```python
from build123d import *

# Parameters (mm, degrees)
SKETCH001_R   = 2.5
SKETCH001_R_2 = 8
PAD_DEPTH     = 1
SKETCH003_R   = 4
PAD001_DEPTH  = 9
SKETCH004_R   = 1.3
POCKET_DEPTH  = 9
FILLET_R      = 10
FILLET001_R   = 15
FILLET002_R   = 30
FILLET003_R   = 10
FILLET004_R   = 10
FILLET005_R   = 5


with BuildPart() as part:
    # Sketch001 → Pad (new body)
    with BuildSketch(Plane.XY):
        Polygon((43.04995, 229.318703), (43.04995, 179.449575), (-116.95005, 179.449575), (-116.95005, 239.449575), (-101.796377, 239.449575), (-91.665504, 229.318703), align=None)
        with Locations((5.54995, 200.560838)):
            Circle(SKETCH001_R, mode=Mode.SUBTRACT)
        with Locations((-99.039165, 191.452072)):
            Circle(SKETCH001_R_2, mode=Mode.SUBTRACT)
        with Locations((30.960835, 191.452072)):
            Circle(SKETCH001_R_2, mode=Mode.SUBTRACT)
        with BuildLine():
            ThreePointArc((25.54995, 206.028969), (20.061493, 220.835101), (5.54995, 227.060838))
            Line((-1.19441, 227.060838), (5.54995, 227.060838))
            Line((-9.694456, 218.560838), (-1.19441, 227.060838))
            Line((-113.95005, 218.561117), (-9.694456, 218.560838))
            Line((-113.95005, 218.561117), (-113.95005, 209.560838))
            Line((-113.95005, 209.560838), (-9.618024, 209.560838))
            Line((-9.618024, 209.560838), (5.54995, 209.560838))
            Line((5.54995, 209.560838), (10.697892, 204.412896))
            Line((10.697892, 189.560838), (10.697892, 204.412896))
            ThreePointArc((10.697892, 189.560838), (21.441031, 194.803313), (25.54995, 206.028969))
        make_face(mode=Mode.SUBTRACT)
        with BuildLine():
            ThreePointArc((-74.793427, 198.14003), (-81.282837, 191.65062), (-74.793427, 185.16121))
            Line((-74.793427, 185.16121), (-26.440948, 185.16121))
            ThreePointArc((-26.440948, 185.16121), (-19.951538, 191.65062), (-26.440948, 198.14003))
            Line((-74.793427, 198.14003), (-26.440948, 198.14003))
        make_face(mode=Mode.SUBTRACT)
    extrude(amount=PAD_DEPTH)

    # Sketch003 (on Face25 of Pad) → Pad001 (join)
    with BuildSketch(Plane.XY.offset(1)):
        with Locations((-104.963402, 231.408722)):
            Circle(SKETCH003_R)
        with Locations((-84.957718, 197.452713)):
            Circle(SKETCH003_R)
    extrude(amount=PAD001_DEPTH)

    # Sketch004 (on Face29 of Pad001) → Pocket (cut)
    with BuildSketch(Plane.XY.offset(10)):
        with Locations((-105.002731, 231.45459)):
            Circle(SKETCH004_R)
        with Locations((-84.991737, 197.493057)):
            Circle(SKETCH004_R)
    extrude(amount=-POCKET_DEPTH, mode=Mode.SUBTRACT)

    # Fillet
    fillet_edges = [part.edges().sort_by_distance(p)[0] for p in [
        (43.04995, 179.449575, 0.5),
    ]]
    fillet(fillet_edges, radius=FILLET_R)

    # Fillet001
    fillet001_edges = [part.edges().sort_by_distance(p)[0] for p in [
        (-116.95005, 179.449575, 0.5),
    ]]
    fillet(fillet001_edges, radius=FILLET001_R)

    # Fillet002
    fillet002_edges = [part.edges().sort_by_distance(p)[0] for p in [
        (43.04995, 229.318703, 0.5),
    ]]
    fillet(fillet002_edges, radius=FILLET002_R)

    # Fillet003
    fillet003_edges = [part.edges().sort_by_distance(p)[0] for p in [
        (-101.796377, 239.449575, 0.5),
    ]]
    fillet(fillet003_edges, radius=FILLET003_R)

    # Fillet004
    fillet004_edges = [part.edges().sort_by_distance(p)[0] for p in [
        (-116.95005, 239.449575, 0.5),
    ]]
    fillet(fillet004_edges, radius=FILLET004_R)

    # Fillet005
    fillet005_edges = [part.edges().sort_by_distance(p)[0] for p in [
        (-91.665504, 229.318703, 0.5),
    ]]
    fillet(fillet005_edges, radius=FILLET005_R)


solid = part.part
```
Could you check a few things on this model? Use its own coordinates, in mm. A direction names the side the tool comes from. Give positions to 0.01 mm unless a question says otherwise; leave off trailing zeros. Loops run counter-clockwise (first coordinate to the right, second up) from the corner with the lowest first, then second, coordinate; pieces in that order, holes last. Notation, with made-up numbers: (55.5, 48.25) - (66.5, 48.25) arc R21 cw to (66.5, 83.25) - close; hole circle Ø11 at (5.25, 1.25). An arc over 180 degrees is marked (long way). Answer in a Markdown table with one row per item. Add a question column.
Q1. Which directions (+Z, -Z, +X, -X, +Y, -Y) give clear straight access to the entire face, cutting with the end or side of a thin tool? Please do faces 4 (the face through (40.2, 182.46, 0.51)), 5 (the face through (8.09, 207.02, 0.49)), 6 (the face through (-105, 231, 1)).
Q2. If we section it at C-C (y = 217): List the corners of the cut face in (x, z) for me.
Q3. If we section it at B-B (z = 6.5): List the corners of the cut face in (x, y) for me.
Q4. If we section it at D-D (x = 19.5): List the corners of the cut face in (y, z) for me.
Q5. For pin 1 (0.5 mm diameter, centred on x = -25, z = 0.5, fed in from +Y); pin 2 (2 mm diameter, centred on x = -84.99, y = 197.49, fed in from +Z); pin 3 (5 mm diameter, centred on y = 197.5, z = 4.5, fed in from -X); pin 4 (6 mm diameter, centred on x = -44.5, y = 193.5, fed in from +Z), each with a flat end and sliding along its axis, tell me the tip position at first contact or that it passes through.
Q6. We'd pull the mould along X, two halves only. Please class faces 1 (the face through (-102.061, 238.667, 0.507)), 2 (the face through (-85.161, 198.782, 5.563)), 3 (the face through (-103, 231, 10)): +X half, -X half, draft (parallel to the pull), parting line (faces both ways), or undercut.
Q7. If we section it at A-A (x = -52): List the corners of the cut face in (y, z) for me.
Q8. Please list where these lines run through material, in increasing order: L1, parallel to Y at x = -40, z = 0.75; L2, parallel to Y at x = 3.5, z = 0.5; L3, parallel to Z at x = -56.5, y = 229. Write a range as from..to.
The answers:
| question | item | result |
|---|---|---|
| 1 | face 4 | +Z, -Z, +X, -Y |
| 1 | face 5 | +Z, -Z |
| 1 | face 6 | +Z |
| 2 | outline | (-116.95, 0) - (-113.95, 0) - (-113.95, 1) - (-116.95, 1) - close; (22.92, 0) - (37.29, 0) - (37.29, 1) - (22.92, 1) - close |
| 3 | outline | circle Ø8 at (-104.96, 231.41); circle Ø8 at (-84.96, 197.45); hole circle Ø2.6 at (-105, 231.45); hole circle Ø2.6 at (-84.99, 197.49) |
| 4 | outline | (179.45, 0) - (192.98, 0) - (192.98, 1) - (179.45, 1) - close; (221.4, 0) - (228.62, 0) - (228.62, 1) - (221.4, 1) - close |
| 5 | pin 1 | stops at y = 229.32 |
| 5 | pin 2 | stops at z = 1 |
| 5 | pin 3 | stops at x = -88.96 |
| 5 | pin 4 | passes through |
| 6 | face 1 | +X half |
| 6 | face 2 | undercut |
| 6 | face 3 | draft |
| 7 | outline | (179.45, 0) - (185.16, 0) - (185.16, 1) - (179.45, 1) - close; (198.14, 0) - (209.56, 0) - (209.56, 1) - (198.14, 1) - close; (218.56, 0) - (229.32, 0) - (229.32, 1) - (218.56, 1) - close |
| 8 | L1 | y = 179.45..185.16, 198.14..209.56, 218.56..229.32 |
| 8 | L2 | y = 179.45..199.13, 201.99..209.56, 227.06..229.32 |
| 8 | L3 | z = 0..1 |
